CAD build for the part. Positions are in the model's coordinates, mm. A direction names the side the tool comes from. Coordinates: 2 decimals unless noted, no trailing zeros. Order: outer loops, then holes, each group sorted by start corner. A loop starts at its lowest first (then second) coordinate and runs counter-clockwise, first axis right, second up. Notation, with made-up numbers: (35, 51) - (73, 51) arc R11 ccw to (73, 66) - close; hole circle Ø2 at (-28, 67). An arc over 180 degrees is marked (long way). Use one line per item in the form item = value.
```python
from build123d import *

# Parameters (mm, degrees)
F0_W     = 49.34406
F0_H     = 94.238028
F1_DEPTH = 76.2
F3_D     = 25.4
F4_R     = 5.08
F5_W     = 20.071493
F5_H     = 6.775275
F6_DEPTH = 25.4


with BuildPart() as f1:
    # F0 (on Top) → F1 (new body)
    with BuildSketch(Plane.XY):
        Rectangle(F0_W, F0_H)
    extrude(amount=F1_DEPTH)

    # F3 (through all)
    with Locations(Plane(origin=(0, 0, 0), x_dir=(1, 0, 0), z_dir=(0, 0, -1))):
        with Locations((0, 0)):
            Hole(F3_D / 2)

    # F4
    f4_edges = [f1.edges().sort_by_distance(p)[0] for p in [
        (0, 47.119014, 0),
        (-24.67203, 0, 0),
        (24.67203, 0, 0),
        (0, -47.119014, 0),
    ]]
    fillet(f4_edges, radius=F4_R)

    # F5 (on face) → F6 (join)
    with BuildSketch(Plane(origin=(0, 0, 0), x_dir=(1, 0, 0), z_dir=(0, 0, -1))):
        with Locations((4.061457, -28.014188)):
            Rectangle(F5_W, F5_H)
    extrude(amount=F6_DEPTH)


solid = f1.part
```
Item 1: Cut at B-B, the plane y = 0. Write the cut outline in (x, z), plus the area to 3 significant figures.
Derived:
outline = (-24.67, 5.08) arc R5.08 ccw to (-19.59, 0) - (-12.7, 0) - (-12.7, 76.2) - (-24.67, 76.2) - close; (12.7, 0) - (19.59, 0) arc R5.08 ccw to (24.67, 5.08) - (24.67, 76.2) - (12.7, 76.2) - close
area = 1,810 mm²
Item 2: Drill centre lines: line 1 (Y direction, x = 0, z = 48); line 2 (Z direction, x = 0.5, y = -33); line 3 (Y direction, x = 6, z = -13.5). Where is each one in solid material? Low to high. Write a range as [from, to].
Derived:
line_1 = [-47.12, -12.7], [12.7, 47.12]
line_2 = [0, 76.2]
line_3 = [24.63, 31.4]
Item 3: Cut at C-C, the plane z = 60. Write the cut outline in (x, y).
Derived:
outline = (-24.67, -47.12) - (24.67, -47.12) - (24.67, 47.12) - (-24.67, 47.12) - close; hole circle Ø25.4 at (0, 0)
Item 4: Cut at D-D, the plane y = 40.5. Write the cut outline in (x, z).
Derived:
outline = (-24.67, 5.08) arc R5.08 ccw to (-19.59, 0) - (19.59, 0) arc R5.08 ccw to (24.67, 5.08) - (24.67, 76.2) - (-24.67, 76.2) - close
Item 5: 3-axis set-ups, long thin cutter, end or side, ignore diameter. For faces 5 (the face through (4, 24.627, -13)), 6 (the face through (-5.974, 28, -13)), 7 (the face through (14.097, 28, -13)), 8 (the face through (4, 31.402, -13)): which of +Z, -Z, +X, -X, +Y, -Y reach the whole face in a straight line?
Derived:
face_5 = -Z, +X, -X, -Y
face_6 = -Z, -X, +Y, -Y
face_7 = -Z, +X, +Y, -Y
face_8 = -Z, +X, -X, +Y
Item 6: Cut at A-A, the plane x = 0. Write the cut outline in (y, z).
Derived:
outline = (-47.12, 5.08) arc R5.08 ccw to (-42.04, 0) - (-12.7, 0) - (-12.7, 76.2) - (-47.12, 76.2) - close; (12.7, 0) - (24.63, 0) - (24.63, -25.4) - (31.4, -25.4) - (31.4, 0) - (42.04, 0) arc R5.08 ccw to (47.12, 5.08) - (47.12, 76.2) - (12.7, 76.2) - close
Item 7: Two-plate mould, pull along X, no slides. Class faces 1 (the face through (2.75, 12.4, 38.63)), 2 (the face through (0, 47.119, 40)), 3 (the face through (-23.223, 0.66, 1.528)), 4 (the face through (23.144, 0.66, 1.449)): +X half, -X half, draft (parallel to the pull), parting line (faces both ways), or undercut.
Derived:
face_1 = undercut
face_2 = draft
face_3 = -X half
face_4 = +X half
Item 8: Drop flat-ended pins along their axis: pin 1 (3.5 mm diameter, centred on y = 28.5, z = -10, fed in from -X); pin 2 (12 mm diameter, centred on x = 12, y = -13, fed in from -Z); pin 3 (1.5 mm diameter, centred on x = -18.5, z = 0.5, fed in from +Y). Give the stop position or say it passes through.
Derived:
pin_1 = -5.97
pin_2 = 0
pin_3 = 45.38
